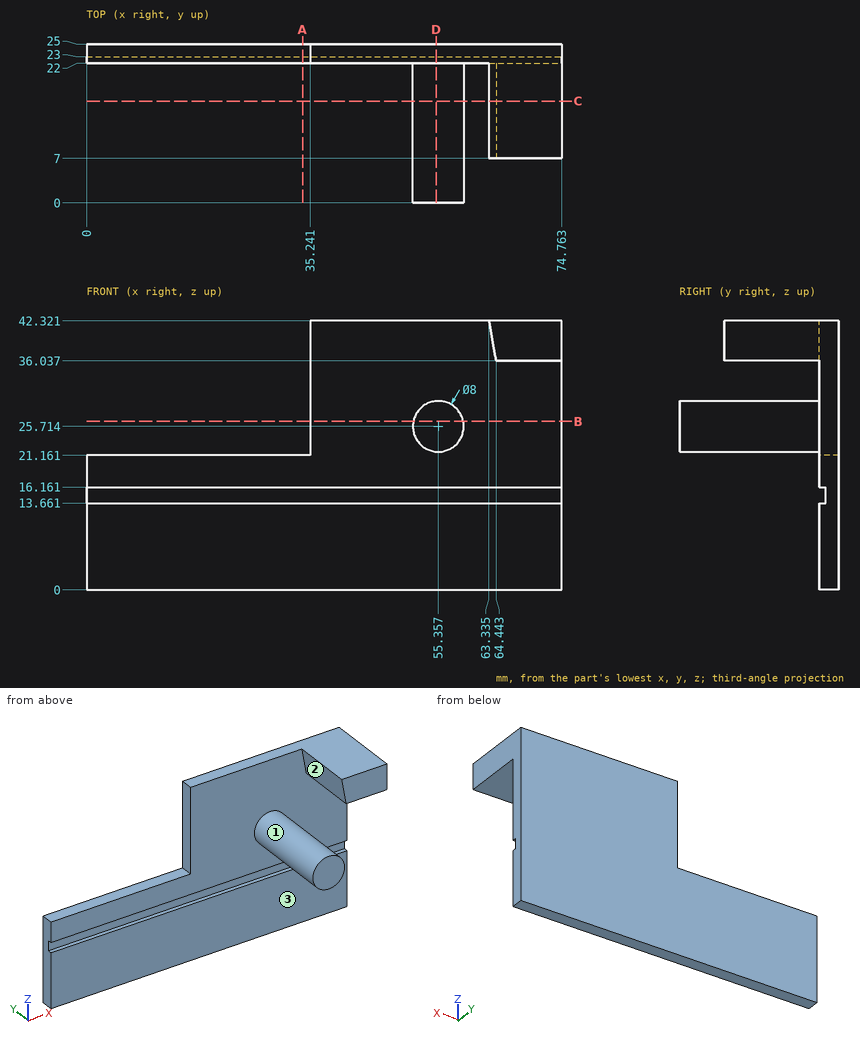
Source: three-view drawing plus pictorial views. Frame: mm from the lowest corner of the part. A direction names the side the tool comes from. Give positions to 0.01 mm unless a question says otherwise; leave off trailing zeros. Order: outer loops, then holes, each group sorted by start corner. A loop starts at its lowest first (then second) coordinate and runs counter-clockwise, first axis right, second up. Notation, with made-up numbers: (4.5, 74.5) -> (43.5, 74.5) arc R16 ccw to (43.5, 85.5) -> close; hole circle Ø11 at (44.25, -34). An arc over 180 degrees is marked (long way). Write each question's results on one line, items separated by ' | '. Start each with the question number.
Item 1: Set-up query: the marked faces 1, 2 and 3. Return all of +Z, -Z, +X, -X, +Y, -Y with unobstructed straight access to the full face (end or side cutting, diameter ignored); none if empty.
Item 2: Contact query for flat-ended pins moving along their axis: P1, Ø5, axis at x = 69, z = 39.5, coming from the -Y side; P2, Ø4, axis at x = 31.5, z = 4, coming from the -Y side; P3, Ø3.5, axis at y = 24, z = 30, coming from the -X side. Output: stop coordinate, or through.
Item 3: Cut plane A-A on x = 34. Return the cut outline in (y, z).
Item 4: Cut plane B-B on z = 26.5. Return the cut outline in (x, y) (1 decimal).
Item 5: Cut plane D-D on x = 55. Return the cut outline in (y, z), then the cut area to 3 significant figures.
Item 6: Line query: line 1 (Y direction, x = 48, z = 7); line 2 (Z direction, x = 69, y = 18.75); line 3 (X direction, y = 17.25, z = 28.5) (1 decimal). Output: solid intervals per line, ascending.
Item 7: Cut plane C-C on y = 16. Return the cut outline in (x, z) (1 decimal).
Established:
1) face 1: -Y | face 2: -Z, -X, -Y | face 3: -Z, +X, -X, -Y
2) P1: y = 7 | P2: y = 22 | P3: x = 35.24
3) outline: (22, 0) -> (25, 0) -> (25, 21.16) -> (22, 21.16) -> (22, 16.16) -> (23, 16.16) -> (23, 13.66) -> (22, 13.66) -> close
4) outline: (35.2, 22) -> (51.4, 22) -> (51.4, 0) -> (59.3, 0) -> (59.3, 22) -> (74.8, 22) -> (74.8, 25) -> (35.2, 25) -> close
5) outline: (0, 21.73) -> (22, 21.73) -> (22, 16.16) -> (23, 16.16) -> (23, 13.66) -> (22, 13.66) -> (22, 0) -> (25, 0) -> (25, 42.32) -> (22, 42.32) -> (22, 29.7) -> (0, 29.7) -> close | area: 300 mm^2
6) line 1: 22 to 25 | line 2: 36.04 to 42.32 | line 3: 52.5 to 58.2
7) outline: circle Ø8 at (55.4, 25.7); (63.3, 42.3) -> (64.4, 36) -> (74.8, 36) -> (74.8, 42.3) -> close
